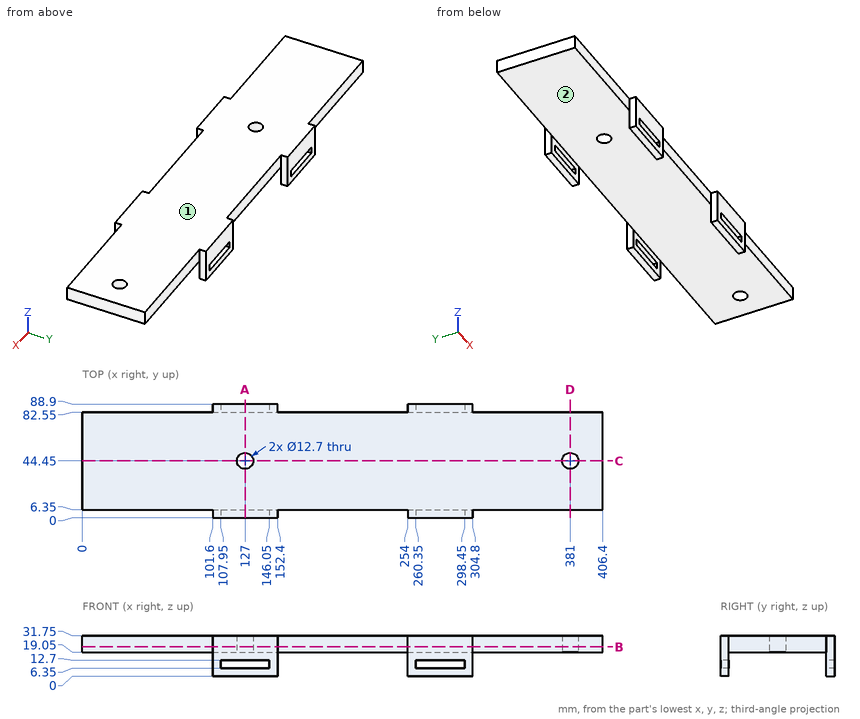
Print and shaded views of the part. All mm, measured from the part's lowest x, y and z. Round coordinates to 2 decimals unless told otherwise and drop trailing zeros. Order: outer loops, then holes, each group sorted by start corner. A loop starts at its lowest first (then second) coordinate and runs counter-clockwise, first axis right, second up.
Q1. Wall check: L1, parallel to X at y = 44, z = 28; L2, parallel to Y at x = 127, z = 23; L3, parallel to Y at x = 151.5, z = 6. Give the ranges that are in metal, low to high.
Q2. Drop flat-ended pins along their axis: pin 1 (1.9 mm diameter, centred on y = 4, z = 10.5, fed in from +X); pin 2 (2 mm diameter, centred on x = 209.5, z = 21.5, fed in from +Y); pin 3 (1 mm diameter, centred on y = 23.5, z = 18, fed in from -X); pin 4 (5 mm diameter, centred on y = 3.5, z = 21, fed in from -X). Give the stop position or say it passes through.
Q3. Slice it at A-A (x = 127). Write the cut outline in (y, z), and give its area (3 significant figures).
Q4. Slice it at B-B (z = 23). Write the cut outline in (x, y), and give its area (3 significant figures).
Q5. Slice it at D-D (x = 381). Write the cut outline in (y, z), and give its area (3 significant figures).
Q6. Slice it at C-C (y = 44.45). Write the cut outline in (x, z), and give its area (3 significant figures).
Q7. Two-plate mould, pull along Y, no slides. Class the marked faces 1 and 2: pulls with the +Y half, pulls with the -Y half, needs draft (parallel to the pull), parting line crosses it, or undercut.
Results below:
1. L1: x = 0 to 120.67, 133.33 to 374.67, 387.33 to 406.4
1. L2: y = 0 to 38.1, 50.8 to 88.9
1. L3: y = 0 to 6.35, 82.55 to 88.9
2. pin 1: stops at x = 304.8
2. pin 2: stops at y = 82.55
2. pin 3: passes through
2. pin 4: stops at x = 101.6
3. outline: (0, 0) - (6.35, 0) - (6.35, 6.35) - (0, 6.35) - close; (0, 12.7) - (6.35, 12.7) - (6.35, 19.05) - (38.1, 19.05) - (38.1, 31.75) - (0, 31.75) - close; (50.8, 19.05) - (82.55, 19.05) - (82.55, 12.7) - (88.9, 12.7) - (88.9, 31.75) - (50.8, 31.75) - close; (82.55, 0) - (88.9, 0) - (88.9, 6.35) - (82.55, 6.35) - close
3. area: 1,130 mm2
4. outline: (0, 6.35) - (101.6, 6.35) - (101.6, 0) - (152.4, 0) - (152.4, 6.35) - (254, 6.35) - (254, 0) - (304.8, 0) - (304.8, 6.35) - (406.4, 6.35) - (406.4, 82.55) - (304.8, 82.55) - (304.8, 88.9) - (254, 88.9) - (254, 82.55) - (152.4, 82.55) - (152.4, 88.9) - (101.6, 88.9) - (101.6, 82.55) - (0, 82.55) - close; hole circle Ø12.7 at (127, 44.45); hole circle Ø12.7 at (381, 44.45)
4. area: 32,000 mm2
5. outline: (6.35, 19.05) - (38.1, 19.05) - (38.1, 31.75) - (6.35, 31.75) - close; (50.8, 19.05) - (82.55, 19.05) - (82.55, 31.75) - (50.8, 31.75) - close
5. area: 806 mm2
6. outline: (0, 19.05) - (120.65, 19.05) - (120.65, 31.75) - (0, 31.75) - close; (133.35, 19.05) - (374.65, 19.05) - (374.65, 31.75) - (133.35, 31.75) - close; (387.35, 19.05) - (406.4, 19.05) - (406.4, 31.75) - (387.35, 31.75) - close
6. area: 4,840 mm2
7. face 1: needs draft
7. face 2: undercut
